Can you work these out from the model? Positions are in its coordinate system, mm. Face numbers are marked on the shaded views. A direction names the side the tool comes from. Coordinates: 2 decimals unless noted, no trailing zeros. Order: outer loops, then holes, each group sorted by start corner. A loop starts at its lowest first (then second) coordinate and runs counter-clockwise, first axis right, second up. Notation, with made-up numbers: (42.25, 42.5) -> (68.25, 42.5) arc R15 ccw to (68.25, 51.5) -> close; hole circle Ø11 at (18, -23). An arc over 180 degrees is marked (long way). Answer as a JSON object with one key per item and string values. Group by question number.
(1) Which directions (+Z, -Z, +X, -X, +Y, -Y) give clear straight access to the entire face, cutting with the end or side of a thin tool? Please do the marked faces 4 and 5.
(2) I need wall thicknesses on line 1 (Y direction, x = 0, z = 11); line 2 (Z direction, x = 12, y = 13.5); line 3 (Z direction, x = 13, y = -24). Which ranges of each line are inside material? Lowest first, please.
(3) I want a section at A-A, the plane y = 0. List the corners of the cut face in (x, z) for me.
(4) For pin 1 (2 mm diameter, centred on x = -4.5, y = 0.5, fed in from +Z); pin 2 (2 mm diameter, centred on x = -13.5, z = 6, fed in from -Y); pin 3 (1 mm diameter, centred on x = -20, z = 11, fed in from +Y), each with a flat end and sliding along its axis, tell me the tip position at first contact or that it passes through.
(5) I want a section at B-B, the plane z = 17. List the corners of the cut face in (x, y) for me, plus the area to 3 significant figures.
(6) If we mould it in two halves opening along X, with no side actions, what happens to the marked faces 1, 2 and 3? For each: pulls with the +X half, pulls with the -X half, needs draft (parallel to the pull), parting line crosses it, or undercut.
from build123d import *

# Parameters (mm, degrees)
SKETCH_1_R          = 30
EXTRUDE_1_DEPTH     = 21
SKETCH_2_R          = 21.15
CUT_EXTRUDE_1_DEPTH = 17


with BuildPart() as part:
    # 草图1 → 凸台-拉伸1 (new body)
    with BuildSketch(Plane.XY):
        with Locations(Location((0, 0, 0), (0, 0, 180))):
            Circle(SKETCH_1_R)
    extrude(amount=EXTRUDE_1_DEPTH)

    # 草图2 → 切除-拉伸1 (cut)
    with BuildSketch(Plane.XY.offset(21)):
        Circle(SKETCH_2_R)
    extrude(amount=-CUT_EXTRUDE_1_DEPTH, mode=Mode.SUBTRACT)

    # 草图4 → 切除-旋转1 (revolve, cut)
    with BuildSketch(Plane(origin=(0, 0, 0), x_dir=(1, 0, 0), z_dir=(0, 1, 0)), mode=Mode.PRIVATE) as cut_revolve_1_sk:
        with BuildLine():
            ThreePointArc((-27, 0), (-29.121320344, -0.878679656), (-30, -3))
            Line((-30, -3), (-30, 0))
            Line((-30, 0), (-27, 0))
        make_face()
        with BuildLine():
            ThreePointArc((-30, -18), (-29.121320344, -20.121320344), (-27, -21))
            Line((-27, -21), (-30, -21))
            Line((-30, -21), (-30, -18))
        make_face()
    revolve(cut_revolve_1_sk.sketch.rotate(Axis((0, 0, 0), (0, 0, -1)), 180), axis=Axis((0, 0, 0), (0, 0, -1)), mode=Mode.SUBTRACT)


solid = part.part
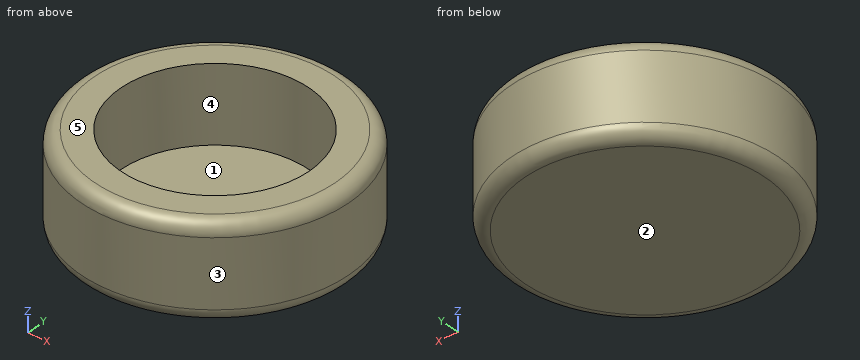
Computed values:
{
 "1": {"face 4": "+Z", "face 5": "+Z, +X, -X, +Y, -Y"},
 "2": {"line 1": "y = -30 to -21.15, 21.15 to 30", "line 2": "z = 0 to 4", "line 3": "z = 0.01 to 20.99"},
 "3": {"outline": "(-30, 3) arc R3 ccw to (-27, 0) -> (27, 0) arc R3 ccw to (30, 3) -> (30, 18) arc R3 ccw to (27, 21) -> (21.15, 21) -> (21.15, 4) -> (-21.15, 4) -> (-21.15, 21) -> (-27, 21) arc R3 ccw to (-30, 18) -> close"},
 "4": {"pin 1": "stops at z = 4", "pin 2": "stops at y = -27.27", "pin 3": "stops at y = 22.8"},
 "5": {"outline": "circle Ø60 at (0, 0); hole circle Ø42.3 at (0, 0)", "area": "1,420 mm2"},
 "6": {"face 1": "undercut", "face 2": "needs draft", "face 3": "parting line crosses it"}
}
